Source: three-view drawing plus pictorial views. Frame: mm from the lowest corner of the part. A direction names the side the tool comes from. Round coordinates to 2 decimals unless told otherwise and drop trailing zeros. Write each loop counter-clockwise with the first axis right and the second up, starting at its lowest first coordinate (ties: lowest second). Pieces come first, ordered by that corner, then holes.
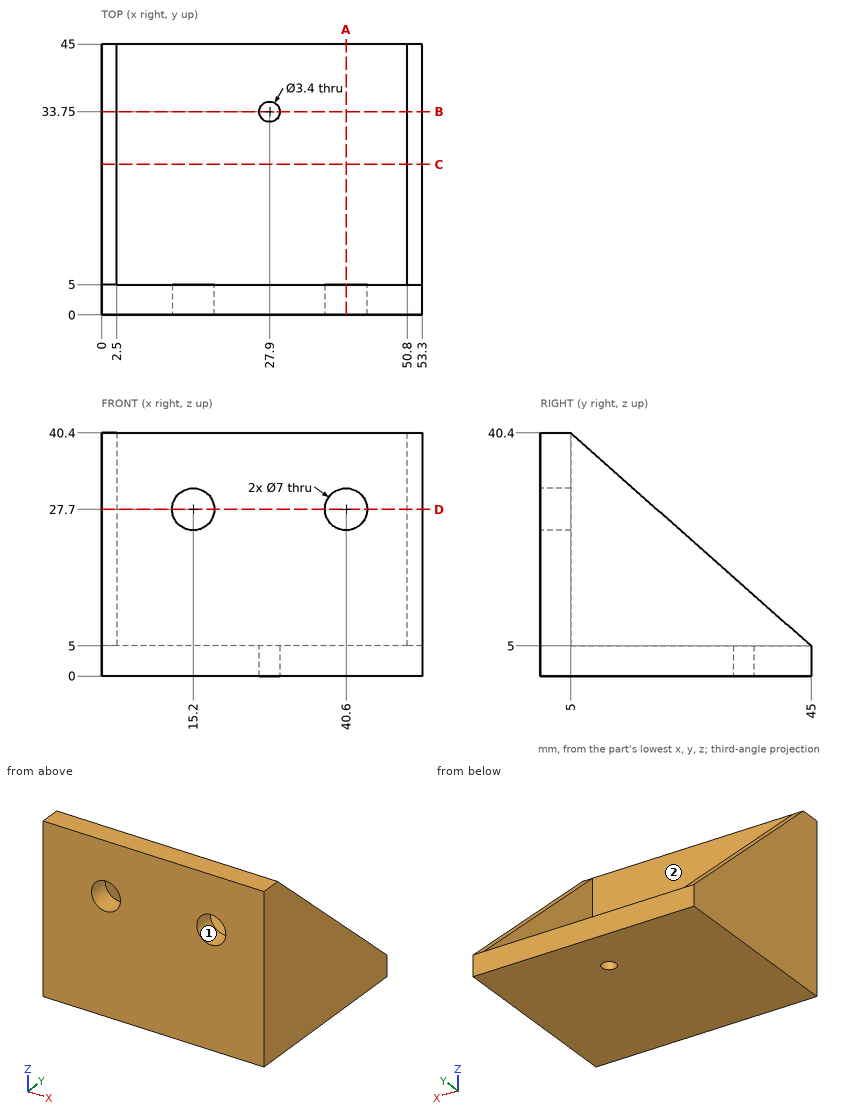
1) Section A-A on x = 40.6. Output: boundary loops of the cut face in (y, z).
2) Reachability of the marked faces 1 and 2 from +Z, -Z, +X, -X, +Y, -Y: full face, straight path, thin tool, end or side. Return the list, or none.
3) Section C-C on y = 25. Output: boundary loops of the cut face in (x, z), plus the area to 3 significant figures.
4) Section B-B on y = 33.75. Output: boundary loops of the cut face in (x, z).
5) Section D-D on z = 27.7. Output: boundary loops of the cut face in (x, y), plus the area to 3 significant figures.
6) Line query: probe 1 along X at (y, z) = (4, 27.7); probe 2 along X at (y, z) = (30, 7); probe 3 along Y at (x, z) = (27.9, 1.1). Output: solid intervals per line, ascending.
7) First-contact query: P1, Ø17.5, axis at x = 30.5, z = 23, coming from the +Y side; P2, Ø4, axis at x = 40.6, z = 27.7, coming from the +Y side; P3, Ø4, axis at x = 27.9, y = 33.75, coming from the +Z side. Flat tips, straight axial feed; report the tip coordinate or a pass-through.
Filled in:
1. outline: (0, 0) - (45, 0) - (45, 5) - (5, 5) - (5, 24.2) - (0, 24.2) - close; (0, 31.2) - (5, 31.2) - (5, 40.4) - (0, 40.4) - close
2. face 1: +Y, -Y
2. face 2: +Z, +Y
3. outline: (0, 0) - (53.3, 0) - (53.3, 22.7) - (50.8, 22.7) - (50.8, 5) - (2.5, 5) - (2.5, 22.7) - (0, 22.7) - close
3. area: 355 mm2
4. outline: (0, 0) - (26.2, 0) - (26.2, 5) - (2.5, 5) - (2.5, 14.96) - (0, 14.96) - close; (29.6, 0) - (53.3, 0) - (53.3, 14.96) - (50.8, 14.96) - (50.8, 5) - (29.6, 5) - close
5. outline: (0, 0) - (11.7, 0) - (11.7, 5) - (2.5, 5) - (2.5, 19.35) - (0, 19.35) - close; (18.7, 0) - (37.1, 0) - (37.1, 5) - (18.7, 5) - close; (44.1, 0) - (53.3, 0) - (53.3, 19.35) - (50.8, 19.35) - (50.8, 5) - (44.1, 5) - close
5. area: 268 mm2
6. probe 1: x = 0 to 11.7, 18.7 to 37.1, 44.1 to 53.3
6. probe 2: x = 0 to 2.5, 50.8 to 53.3
6. probe 3: y = 0 to 32.05, 35.45 to 45
7. P1: stops at y = 5
7. P2: passes through
7. P3: stops at z = 5
